Here's how the part is built. I have some questions about the finished solid (model axes, mm). A direction names the side the tool comes from. Coordinates: 2 decimals unless noted, no trailing zeros. Loops run counter-clockwise (first coordinate to the right, second up) from the corner with the lowest first, then second, coordinate; pieces in that order, holes last. Notation, with made-up numbers: (4, -39.75) -> (61, -39.75) arc R5 cw to (61, -34.75) -> close; hole circle Ø8 at (15, 21.25). An arc over 180 degrees is marked (long way). Answer as a JSON object with one key per item and string values. Group by question number.
Q1. Thinking about a two-plate mould opening in X: for faces 6 (the cylindrical face through (-99.859, 10.203, 1.972)), 7 (the cylindrical face through (108.859, 63.797, 21.72)), 8 (the flat face through (54, -9, 2)), 9 (the flat face through (-107, 40.5, 10)), which applies, released by +X, released by -X, zero draft, split by the parting line, or undercut?
Q2. I want a section at A-A on z = 19. Write out the boundary of the cut face in (x, y), then the cut area to 3 significant figures.
Q3. I'm going to push flat-ended pins straight in: pin 1 (1.7 mm diameter, centred on y = -47.5, z = 9, fed in from -X); pin 2 (2 mm diameter, centred on y = 31.5, z = 1.5, fed in from +X); pin 3 (4.5 mm diameter, centred on x = -107, z = 10, fed in from -Y); pin 4 (3.5 mm diameter, centred on x = 104.5, z = 16.5, fed in from -Y). Where does each tip first touch, or does it pass through?
Q4. I want a section at B-B on x = -1. Write out the boundary of the cut face in (y, z).
Q5. On a 3-axis mill with a long thin cutter (end or side, diameter ignored), from which of +Z, -Z, +X, -X, +Y, -Y can I reach the whole of each face in a straight line? I mean faces 1 (the flat face through (1, 19, 0)), 2 (the flat face through (-107, 54.5, 10)), 3 (the cylindrical face through (99.859, 54.797, 1.972)), 4 (the flat face through (107, 30, 42)), 5 (the flat face through (107, -5, 23)). Say none if no direction works.
Q6. I need wall thicknesses on line 1 (Z direction, x = 105.45, y = 4); line 2 (X direction, y = 50, z = 8); line 3 (X direction, y = 39.5, z = 12). Which ranges of each line are inside material? Lowest first, please.
```python
from build123d import *

# Parameters (mm, degrees)
PAD_DEPTH       = 4
PAD001_DEPTH    = 38
SKETCH007_R     = 1.4
POCKET_DEPTH    = 8
PAD002_DEPTH    = 12
SKETCH009_R     = 1.4
POCKET001_DEPTH = 8
PAD003_DEPTH    = 28
SKETCH011_W     = 9
SKETCH011_H     = 1.7
POCKET002_DEPTH = 5
FILLET_R        = 2


with BuildPart() as part:
    # Sketch → Pad (new body)
    with BuildSketch(Plane.XY):
        with BuildLine():
            Line((-106, 65), (106, 65))
            ThreePointArc((110, 61), (108.828427, 63.828427), (106, 65))
            Line((110, 61), (110, -61))
            ThreePointArc((106, -65), (108.828427, -63.828427), (110, -61))
            Line((106, -65), (-106, -65))
            ThreePointArc((-110, -61), (-108.828427, -63.828427), (-106, -65))
            Line((-110, -61), (-110, 61))
            ThreePointArc((-106, 65), (-108.828427, 63.828427), (-110, 61))
        make_face()
        with BuildLine():
            ThreePointArc((13, -9), (10.171573, -10.171573), (9, -13))
            Line((9, -53), (9, -13))
            ThreePointArc((9, -53), (10.171573, -55.828427), (13, -57))
            Line((97, -57), (13, -57))
            ThreePointArc((97, -57), (99.828427, -55.828427), (101, -53))
            Line((101, -13), (101, -53))
            ThreePointArc((101, -13), (99.828427, -10.171573), (97, -9))
            Line((13, -9), (97, -9))
        make_face(mode=Mode.SUBTRACT)
        with BuildLine():
            ThreePointArc((13, 56), (10.171573, 54.828427), (9, 52))
            Line((9, 13), (9, 52))
            ThreePointArc((9, 13), (10.171573, 10.171573), (13, 9))
            Line((97, 9), (13, 9))
            ThreePointArc((97, 9), (99.828427, 10.171573), (101, 13))
            Line((101, 52), (101, 13))
            ThreePointArc((101, 52), (99.828427, 54.828427), (97, 56))
            Line((13, 56), (97, 56))
        make_face(mode=Mode.SUBTRACT)
        with BuildLine():
            ThreePointArc((-97, 56), (-99.828427, 54.828427), (-101, 52))
            Line((-101, 13), (-101, 52))
            ThreePointArc((-101, 13), (-99.828427, 10.171573), (-97, 9))
            Line((-13, 9), (-97, 9))
            ThreePointArc((-13, 9), (-10.171573, 10.171573), (-9, 13))
            Line((-9, 52), (-9, 13))
            ThreePointArc((-9, 52), (-10.171573, 54.828427), (-13, 56))
            Line((-97, 56), (-13, 56))
        make_face(mode=Mode.SUBTRACT)
        with BuildLine():
            ThreePointArc((-97, -9), (-99.828427, -10.171573), (-101, -13))
            Line((-101, -52), (-101, -13))
            ThreePointArc((-101, -52), (-99.828427, -54.828427), (-97, -56))
            Line((-13, -56), (-97, -56))
            ThreePointArc((-13, -56), (-10.171573, -54.828427), (-9, -52))
            Line((-9, -13), (-9, -52))
            ThreePointArc((-9, -13), (-10.171573, -10.171573), (-13, -9))
            Line((-97, -9), (-13, -9))
        make_face(mode=Mode.SUBTRACT)
    extrude(amount=PAD_DEPTH)

    # Sketch006 (on Face42 of Pad) → Pad001 (join)
    with BuildSketch(Plane.XY.offset(4)):
        with BuildLine():
            ThreePointArc((105, 65), (104.292893, 64.707107), (104, 64))
            Line((104, -4), (104, 64))
            ThreePointArc((104, -4), (104.292893, -4.707107), (105, -5))
            Line((109, -5), (105, -5))
            ThreePointArc((109, -5), (109.707107, -4.707107), (110, -4))
            Line((110, 61), (110, -4))
            ThreePointArc((110, 61), (108.828427, 63.828427), (106, 65))
            Line((105, 65), (106, 65))
        make_face()
    extrude(amount=PAD001_DEPTH)

    # Sketch007 (on Face50 of Pad001) → Pocket (cut)
    with BuildSketch(Plane.YZ.offset(110)):
        with Locations((56, 36)):
            Circle(SKETCH007_R)
        with Locations((4, 36)):
            Circle(SKETCH007_R)
    extrude(amount=-POCKET_DEPTH, mode=Mode.SUBTRACT)

    # Sketch008 (on Face5 of Pocket) → Pad002 (join)
    with BuildSketch(Plane.XY.offset(4)):
        with BuildLine():
            ThreePointArc((-109, 54.5), (-109.707107, 54.207107), (-110, 53.5))
            Line((-110, 41.5), (-110, 53.5))
            ThreePointArc((-110, 41.5), (-109.707107, 40.792893), (-109, 40.5))
            Line((-105, 40.5), (-109, 40.5))
            ThreePointArc((-105, 40.5), (-104.292893, 40.792893), (-104, 41.5))
            Line((-104, 53.5), (-104, 41.5))
            ThreePointArc((-104, 53.5), (-104.292893, 54.207107), (-105, 54.5))
            Line((-109, 54.5), (-105, 54.5))
        make_face()
        with BuildLine():
            ThreePointArc((-109, -40.5), (-109.707107, -40.792893), (-110, -41.5))
            Line((-110, -53.5), (-110, -41.5))
            ThreePointArc((-110, -53.5), (-109.707107, -54.207107), (-109, -54.5))
            Line((-105, -54.5), (-109, -54.5))
            ThreePointArc((-105, -54.5), (-104.292893, -54.207107), (-104, -53.5))
            Line((-104, -41.5), (-104, -53.5))
            ThreePointArc((-104, -41.5), (-104.292893, -40.792893), (-105, -40.5))
            Line((-109, -40.5), (-105, -40.5))
        make_face()
    extrude(amount=PAD002_DEPTH)

    # Sketch009 (on Face7 of Pad002) → Pocket001 (cut)
    with BuildSketch(Plane(origin=(-110, 0, 0), x_dir=(0, -1, 0), z_dir=(-1, 0, 0))):
        with Locations((-47.5, 9)):
            Circle(SKETCH009_R)
        with Locations((47.5, 9)):
            Circle(SKETCH009_R)
    extrude(amount=-POCKET001_DEPTH, mode=Mode.SUBTRACT)

    # Sketch010 (on Face5 of Pocket001) → Pad003 (join)
    with BuildSketch(Plane.XY.offset(4)):
        with BuildLine():
            ThreePointArc((102, -13.95), (101.292893, -14.242893), (101, -14.95))
            Line((101, -28.65), (101, -14.95))
            ThreePointArc((101, -28.65), (101.292893, -29.357107), (102, -29.65))
            Line((109, -29.65), (102, -29.65))
            ThreePointArc((109, -29.65), (109.707107, -29.357107), (110, -28.65))
            Line((110, -14.95), (110, -28.65))
            ThreePointArc((110, -14.95), (109.707107, -14.242893), (109, -13.95))
            Line((102, -13.95), (109, -13.95))
        make_face()
    extrude(amount=PAD003_DEPTH)

    # Sketch011 (on Face82 of Pad003) → Pocket002 (cut)
    with BuildSketch(Plane.XY.offset(32)):
        with Locations((105.5, -21.8)):
            Rectangle(SKETCH011_W, SKETCH011_H)
    extrude(amount=-POCKET002_DEPTH, mode=Mode.SUBTRACT)

    # Fillet
    fillet_edges = [part.edges().sort_by_distance(p)[0] for p in [
        (0, 65, 0),
    ]]
    fillet(fillet_edges, radius=FILLET_R)


solid = part.part
```
Result set:
{
 "1": {"face 6": "undercut", "face 7": "released by +X", "face 8": "undercut", "face 9": "zero draft"},
 "2": {"outline": "(101, -28.65) arc R1 ccw to (102, -29.65) -> (109, -29.65) arc R1 ccw to (110, -28.65) -> (110, -14.95) arc R1 ccw to (109, -13.95) -> (102, -13.95) arc R1 ccw to (101, -14.95) -> close; (104, -4) arc R1 ccw to (105, -5) -> (109, -5) arc R1 ccw to (110, -4) -> (110, 61) arc R4 ccw to (106, 65) -> (105, 65) arc R1 ccw to (104, 64) -> close", "area": "556 mm²"},
 "3": {"pin 1": "passes through", "pin 2": "stops at x = 110", "pin 3": "stops at y = -54.5", "pin 4": "stops at y = -29.65"},
 "4": {"outline": "(-65, 2) arc R2 ccw to (-63, 0) -> (63, 0) arc R2 ccw to (65, 2) -> (65, 4) -> (-65, 4) -> close"},
 "5": {"face 1": "-Z, +X, -X, +Y, -Y", "face 2": "+Z, -X, +Y", "face 3": "+Z, -Z", "face 4": "+Z, +X, -X, +Y, -Y", "face 5": "+Z, +X, -X"},
 "6": {"line 1": "z = 0 to 34.6, 37.4 to 42", "line 2": "x = -110 to -104, 104 to 110", "line 3": "x = 104 to 110"}
}
